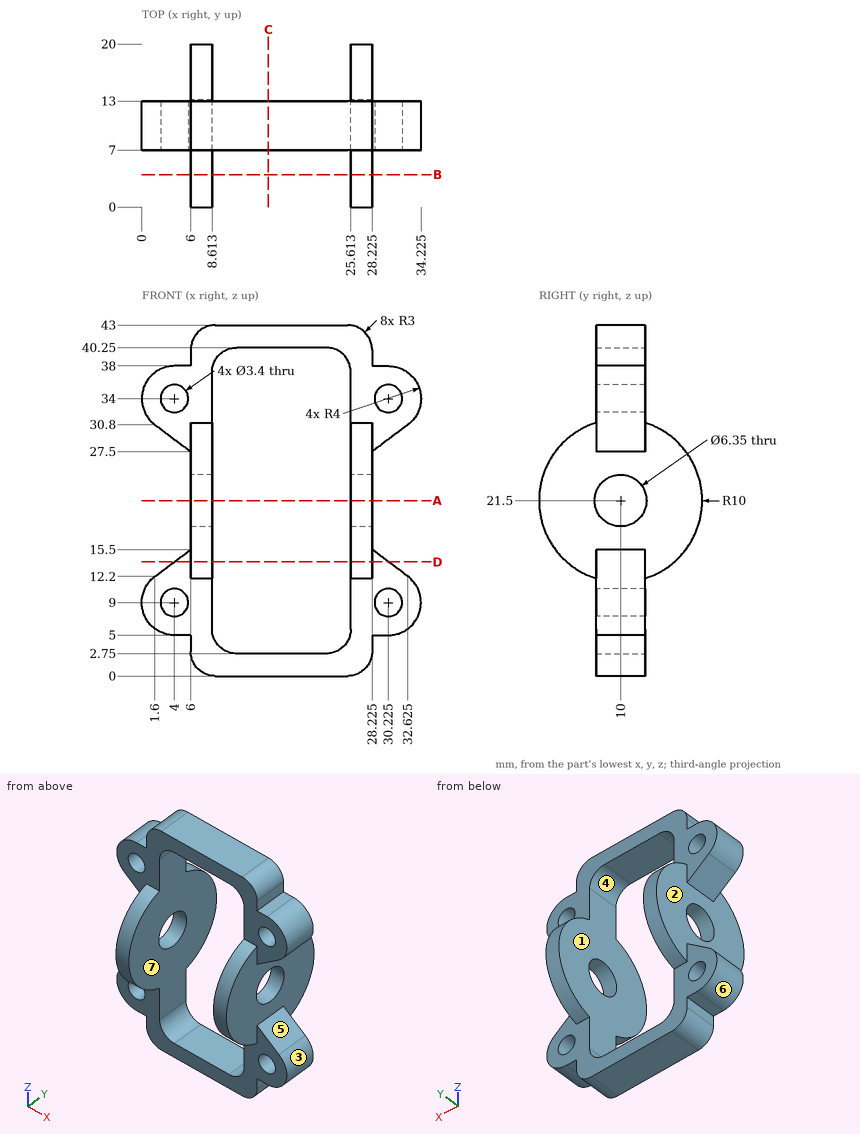
The figure shows three views and two pictorial views of one solid part (mm, origin at its lowest corner). Answer the questions. A direction names the side the tool comes from. Round coordinates to 2 decimals unless told otherwise and drop trailing zeros. Loops run counter-clockwise (first coordinate to the right, second up) from the corner with the lowest first, then second, coordinate; pieces in that order, holes last. Notation, with made-up numbers: (-23, 44) - (15, 44) arc R23 cw to (15, 66) - close; hole circle Ø5 at (12.25, 18.25). An arc over 180 degrees is marked (long way). Use one line per item in the form item = value. Start each with the question number.
(1) Flat-ended cylindrical pins translate along their axes: P1, Ø1.5, axis at y = 12, z = 16, coming from the -X side (1 decimal); P2, Ø5, axis at y = 9.5, z = 25.5, coming from the +X side; P3, Ø17, axis at x = 14, z = 5, coming from the -Y side; P4, Ø2.5, axis at x = 30.225, z = 34, coming from the -Y side. Find the tip coordinate at first contact, or state that the pin passes through.
(2) Determine the mould class of the marked faces 1, 2, 3 and 4 for opening direction X: +X half, -X half, draft (parallel to the pull), parting line (faces both ways), or undercut.
(3) Find section A-A on z = 21.5. Determine the outline of the cut face in (x, y) (1 decimal).
(4) Find section B-B on y = 4. Determine the outline of the cut face in (x, z) (1 decimal).
(5) Which of the six approach directions +Z, -Z, +X, -X, +Y, -Y give full straight-line access (tool end or side, diameter ignored) to the marked faces 5, 6 and 7?
(6) Find section D-D on z = 14. Determine the outline of the cut face in (x, y) (1 decimal).
(7) Find section C-C on x = 15.5. Determine the outline of the cut face in (y, z).
(8) Consider line 1 (X direction, y = 11.35, z = 34) (1 decimal); line 2 (X direction, y = 6.75, z = 12.5) (1 decimal); line 3 (Y direction, x = 6.9, z = 21.5) (1 decimal). Determine where each line is inside the solid, lowest interval first.
Answer list:
q1.P1 = 5.7
q1.P2 = 28.89
q1.P3 = 7
q1.P4 = through
q2.face_1 = undercut
q2.face_2 = -X half
q2.face_3 = +X half
q2.face_4 = undercut
q3.outline = (6, 0) - (8.6, 0) - (8.6, 6.8) - (6, 6.8) - close; (6, 13.2) - (8.6, 13.2) - (8.6, 20) - (6, 20) - close; (25.6, 0) - (28.2, 0) - (28.2, 6.8) - (25.6, 6.8) - close; (25.6, 13.2) - (28.2, 13.2) - (28.2, 20) - (25.6, 20) - close
q4.outline = (6, 13.5) - (8.6, 13.5) - (8.6, 29.5) - (6, 29.5) - close; (25.6, 13.5) - (28.2, 13.5) - (28.2, 29.5) - (25.6, 29.5) - close
q5.face_5 = +X, +Y, -Y
q5.face_6 = -X, +Y, -Y
q5.face_7 = +Y, -Y
q6.outline = (4, 7) - (6, 7) - (6, 3.4) - (8.6, 3.4) - (8.6, 16.6) - (6, 16.6) - (6, 13) - (4, 13) - close; (25.6, 3.4) - (28.2, 3.4) - (28.2, 7) - (30.2, 7) - (30.2, 13) - (28.2, 13) - (28.2, 16.6) - (25.6, 16.6) - close
q7.outline = (7, 0) - (13, 0) - (13, 2.75) - (7, 2.75) - close; (7, 40.25) - (13, 40.25) - (13, 43) - (7, 43) - close
q8.line_1 = 0 to 2.3, 5.7 to 8.6, 25.6 to 28.5, 31.9 to 34.2
q8.line_2 = 6 to 8.6, 25.6 to 28.2
q8.line_3 = 0 to 6.8, 13.2 to 20
